Geometry check sheet. Reference: drawing and pictorial views, mm from the part's lowest x, y, z. A direction names the side the tool comes from. Give positions to 0.01 mm unless a question says otherwise; leave off trailing zeros. Order: outer loops, then holes, each group sorted by start corner. A loop starts at its lowest first (then second) coordinate and runs counter-clockwise, first axis right, second up.
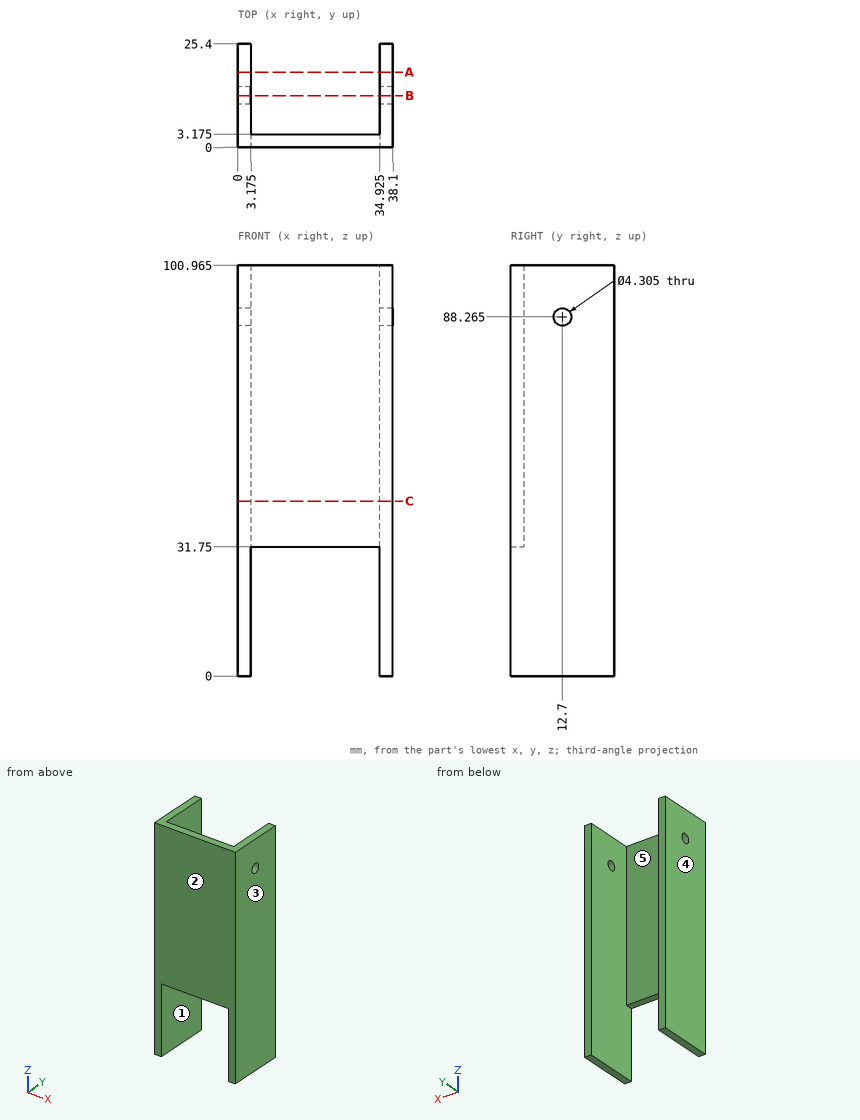
(1) Cross-section at C-C on z = 43. Enter the section's corners in (x, y) (1 decimal).
Response values:
outline: (0, 0) - (38.1, 0) - (38.1, 25.4) - (34.9, 25.4) - (34.9, 3.2) - (3.2, 3.2) - (3.2, 25.4) - (0, 25.4) - close
(2) Cross-section at B-B on y = 12.7. Enter the section's corners in (x, z) (1 decimal).
Response values:
outline: (0, 0) - (3.2, 0) - (3.2, 86.1) - (0, 86.1) - close; (0, 90.4) - (3.2, 90.4) - (3.2, 101) - (0, 101) - close; (34.9, 0) - (38.1, 0) - (38.1, 86.1) - (34.9, 86.1) - close; (34.9, 90.4) - (38.1, 90.4) - (38.1, 101) - (34.9, 101) - close
(3) Gauge pin test, flat ends, axial feed: pin 1 Ø4 at (y, z) = (12.7, 88.265) entering from -X; pin 2 Ø1 at (x, y) = (13.5, 1) entering from -Z. Record the tip position at first contact, or that the pin passes through.
Response values:
pin 1: passes through
pin 2: stops at z = 31.75
(4) Release check for a two-part mould opening along X. For the marked faces 1, 2 and 3 record: released by +X, released by -X, zero draft, split by the parting line, or undercut.
Response values:
face 1: undercut
face 2: zero draft
face 3: released by +X
(5) Set-up check for the marked faces 4 and 5: record each of +Z, -Z, +X, -X, +Y, -Y from which the full face is reachable in a straight line by a thin tool's end or side.
Response values:
face 4: +Z, -Z, -X, +Y, -Y
face 5: +Z, -Z, +Y
(6) Material ranges on L1, parallel to X at y = 17.5, z = 96.5 (1 decimal); L2, parallel to Y at x = 33.5, z = 64.5 (1 decimal), recorded low to high.
Response values:
L1: x = 0 to 3.2, 34.9 to 38.1
L2: y = 0 to 3.2
(7) Cross-section at A-A on y = 18.5. Enter the section's corners in (x, z) (1 decimal), then the cut area to 3 significant figures.
Response values:
outline: (0, 0) - (3.2, 0) - (3.2, 101) - (0, 101) - close; (34.9, 0) - (38.1, 0) - (38.1, 101) - (34.9, 101) - close
area: 641 mm2
